from build123d import *

# Parameters (mm, degrees)
F0_W     = 63.5
F0_H     = 50.8
F1_DEPTH = 63.5
F2_W     = 12.7
F2_H     = 50.8
F3_DEPTH = 25.4
F2_W_2   = 25.4
F2_H_2   = 25.4
F4_DEPTH = 25.4


with BuildPart() as f1:
    # F0 (on Front) → F1 (new body)
    with BuildSketch(Plane.XZ):
        with Locations((-9.895136, -14.676312)):
            Rectangle(F0_W, F0_H)
    extrude(amount=F1_DEPTH)

    # F2 (on face) → F3 (cut)
    with BuildSketch(Plane.XY.offset(10.723688)):
        with Locations((-22.595136, -38.1)):
            Rectangle(F2_W, F2_H)
    extrude(amount=-F3_DEPTH, mode=Mode.SUBTRACT)

    # F2 (on face) → F4 (cut)
    with BuildSketch(Plane.XY.offset(10.723688)):
        with Locations((9.154864, -25.4)):
            Rectangle(F2_W_2, F2_H_2)
    extrude(amount=-F4_DEPTH, mode=Mode.SUBTRACT)


solid = f1.part
Input: part model. Units: mm. Frame: model coordinates. A direction names the side the tool comes from. Round coordinates to 2 decimals unless told otherwise and drop trailing zeros. Order: outer loops, then holes, each group sorted by start corner. A loop starts at its lowest first (then second) coordinate and runs counter-clockwise, first axis right, second up. Notation, with made-up numbers: (32, 80) - (69, 80) arc R22 ccw to (69, 101) - close; hole circle Ø8 at (-25, -33.5). An arc over 180 degrees is marked (long way). Use a Markdown table: item, result.
1. Mould query, pull axis Y, two halves, no side actions, for faces 1 (the face through (9, -25, -14.676)), 2 (the face through (-23, -38, -14.676)), 3 (the face through (-10, 0, -14)), 4 (the face through (-10, -63.5, -14)). Classes: +Y half, -Y half, draft (parallel to the pull), parting line (faces both ways), or undercut.
Evaluation:
| item | result |
|---|---|
| face 1 | undercut |
| face 2 | draft |
| face 3 | +Y half |
| face 4 | -Y half |
2. Material intervals for probe 1 along X at (y, z) = (-58.5, 3); probe 2 along Y at (x, z) = (6.5, 4); probe 3 along X at (y, z) = (-37, -2), sorted ascending.
Evaluation:
| item | result |
|---|---|
| probe 1 | -41.65 to -28.95, -16.25 to 21.85 |
| probe 2 | -63.5 to -38.1, -12.7 to 0 |
| probe 3 | -41.65 to -28.95, -16.25 to -3.55 |
3. Access query for faces 5 (the face through (-16.245, -38, -2)), 6 (the face through (-3.545, -26, -2)), 7 (the face through (-10, -31, -40.076)). Directions: +Z, -Z, +X, -X, +Y, -Y. A direction counts if a zero-diameter tool reaches every point of the face in a straight line with its end or side. Return the directions, or none.
Evaluation:
| item | result |
|---|---|
| face 5 | +Z, -Y |
| face 6 | +Z, +X |
| face 7 | -Z, +X, -X, +Y, -Y |
4. First-contact query: pin 1 (14 mm diameter, centred on x = -25, y = -37, fed in from +Z); pin 2 (2 mm diameter, centred on y = -21, z = -2.5, fed in from +X); pin 3 (20.5 mm diameter, centred on x = 9.5, y = -24.5, fed in from +Z). Flat tips, straight axial feed; report the tip coordinate or a pass-through.
Evaluation:
| item | result |
|---|---|
| pin 1 | z = 10.72 |
| pin 2 | x = -3.55 |
| pin 3 | z = -14.68 |
5. Section B-B on z = -5. Return the cut outline in (x, y).
Evaluation:
| item | result |
|---|---|
| outline | (-41.65, -63.5) - (-28.95, -63.5) - (-28.95, -12.7) - (-16.25, -12.7) - (-16.25, -63.5) - (21.85, -63.5) - (21.85, -38.1) - (-3.55, -38.1) - (-3.55, -12.7) - (21.85, -12.7) - (21.85, 0) - (-41.65, 0) - close |
6. Section C-C on y = -17.5. Return the cut outline in (x, z).
Evaluation:
| item | result |
|---|---|
| outline | (-41.65, -40.08) - (21.85, -40.08) - (21.85, -14.68) - (-3.55, -14.68) - (-3.55, 10.72) - (-16.25, 10.72) - (-16.25, -14.68) - (-28.95, -14.68) - (-28.95, 10.72) - (-41.65, 10.72) - close |
7. Section A-A on y = -52.5. Return the cut outline in (x, z), then the cut area to 3 significant figures.
Evaluation:
| item | result |
|---|---|
| outline | (-41.65, -40.08) - (21.85, -40.08) - (21.85, 10.72) - (-16.25, 10.72) - (-16.25, -14.68) - (-28.95, -14.68) - (-28.95, 10.72) - (-41.65, 10.72) - close |
| area | 2,900 mm^2 |
